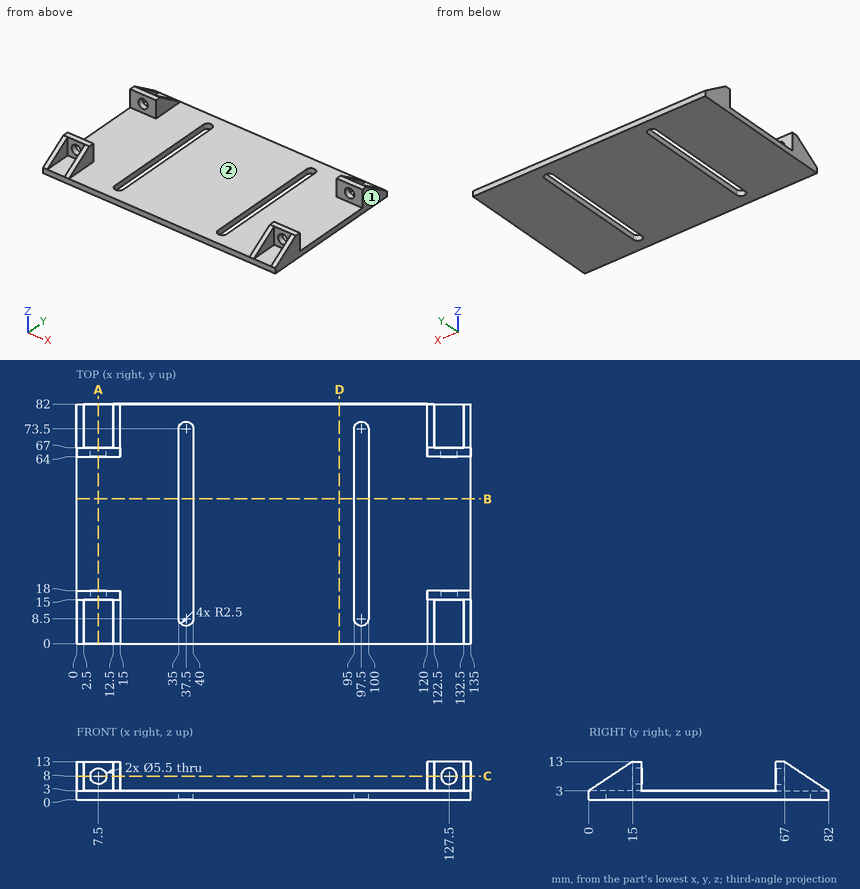
Check sheet for the drawn part. Datum: minimum x, y, z corner. Units: mm. Round coordinates to 2 decimals unless told otherwise and drop trailing zeros. Loops run counter-clockwise (first coordinate to the right, second up) from the corner with the lowest first, then second, coordinate; pieces in that order, holes last. Notation, with made-up numbers: (31.5, 82.25) -> (64.5, 82.25) arc R8 ccw to (64.5, 93.25) -> close; hole circle Ø11 at (-21, 2.25). An arc over 180 degrees is marked (long way). Put each result on its own line as item: value. Start each with the question number.
1. Scan lines: probe 1 along Z at (x, y) = (7.5, 65.6); probe 2 along Z at (x, y) = (116, 64); probe 3 along Y at (x, z) = (123, 10.5). Record each from-to range of solid material in increasing order.
2. Section check A-A (x = 7.5). Enter the section's corners in (y, z), plus the area to 3 significant figures.
3. Section check B-B (y = 49.5). Enter the section's corners in (x, z), plus the area to 3 significant figures.
4. Gauge pin test, flat ends, axial feed: pin 1 (5 mm diameter, centred on x = 7.5, z = 8, fed in from -Y); pin 2 (4 mm diameter, centred on x = 86.5, y = 26, fed in from +Z). Record the tip position at first contact, or that the pin passes through.
5. Draft check along Y on the marked faces 1 and 2. Enter one of: +Y half, -Y half, draft (parallel to the pull), parting line (faces both ways), or undercut.
6. Section check D-D (x = 90). Enter the section's corners in (y, z).
7. Section check C-C (z = 8). Give the number of separate pieces and of enclosed holes in the cut face, plus the area to 3 significant figures.
Findings:
1. probe 1: z = 0 to 5.25, 10.75 to 13
1. probe 2: z = 0 to 3
1. probe 3: y = 15 to 18, 64 to 67
2. outline: (0, 0) -> (82, 0) -> (82, 3) -> (67, 3) -> (67, 5.25) -> (64, 5.25) -> (64, 3) -> (18, 3) -> (18, 5.25) -> (15, 5.25) -> (15, 3) -> (0, 3) -> close; (15, 10.75) -> (18, 10.75) -> (18, 13) -> (15, 13) -> close; (64, 10.75) -> (67, 10.75) -> (67, 13) -> (64, 13) -> close
2. area: 273 mm^2
3. outline: (0, 0) -> (35, 0) -> (35, 3) -> (0, 3) -> close; (40, 0) -> (95, 0) -> (95, 3) -> (40, 3) -> close; (100, 0) -> (135, 0) -> (135, 3) -> (100, 3) -> close
3. area: 375 mm^2
4. pin 1: passes through
4. pin 2: stops at z = 3
5. face 1: draft
5. face 2: undercut
6. outline: (0, 0) -> (82, 0) -> (82, 3) -> (0, 3) -> close
7. separate pieces: 8
7. enclosed holes: 0
7. area: 264 mm^2
